Check sheet for the modelled part. Datum: model origin and axes. Units: mm. Give positions to 0.01 mm unless a question says otherwise; leave off trailing zeros. Order: outer loops, then holes, each group sorted by start corner. A loop starts at its lowest first (then second) coordinate and runs counter-clockwise, first axis right, second up.
```python
from build123d import *

# Parameters (mm, degrees)
EXTRUDE_1_DEPTH      = 3
EXTRUDE_1_DEPTH_BACK = 6
SKETCH_2_R           = 60
SKETCH_5_R           = 4
EXTRUDE_2_DEPTH      = 112
SKETCH_6_R           = 4
EXTRUDE_3_DEPTH      = 112
SKETCH_7_R           = 13
CUT_EXTRUDE_2_DEPTH  = 20
SKETCH_14_W          = 26
SKETCH_14_H          = 65
CUT_EXTRUDE_3_DEPTH  = 10


with BuildPart() as part:
    # 草图2 → 凸台-拉伸1 (new, two sides: drawn at the far end of the back side and taken through both)
    with BuildSketch(Plane.XY.offset(-EXTRUDE_1_DEPTH_BACK)):
        Circle(SKETCH_2_R)
    extrude(amount=EXTRUDE_1_DEPTH + EXTRUDE_1_DEPTH_BACK)

    # 草图5 → 凸台-拉伸2 (add)
    with BuildSketch(Plane(origin=(0, 0, -6), x_dir=(-1, 0, 0), z_dir=(0, 0, -1))):
        with Locations(Location((0, 50, 0), (0, 0, 180))):
            Circle(SKETCH_5_R)
    extrude(amount=EXTRUDE_2_DEPTH)

    # 草图6 → 凸台-拉伸3 (add)
    with BuildSketch(Plane(origin=(0, 0, -6), x_dir=(-1, 0, 0), z_dir=(0, 0, -1))):
        with Locations(Location((-44.655818583, -22.491284238, 0), (0, 0, 180))):
            Circle(SKETCH_6_R)
        with Locations(Location((41.95168902, -27.203966409, 0), (0, 0, 180))):
            Circle(SKETCH_6_R)
    extrude(amount=EXTRUDE_3_DEPTH)

    # 草图7 → 切除-拉伸2 (cut)
    with BuildSketch(Plane.XY.offset(3)):
        Circle(SKETCH_7_R)
    extrude(amount=-CUT_EXTRUDE_2_DEPTH, mode=Mode.SUBTRACT)

    # 草图14 → 切除-拉伸3 (cut)
    with BuildSketch(Plane.XY.offset(3)):
        with Locations((0, -32.5)):
            Rectangle(SKETCH_14_W, SKETCH_14_H)
    extrude(amount=-CUT_EXTRUDE_3_DEPTH, mode=Mode.SUBTRACT)


solid = part.part
```
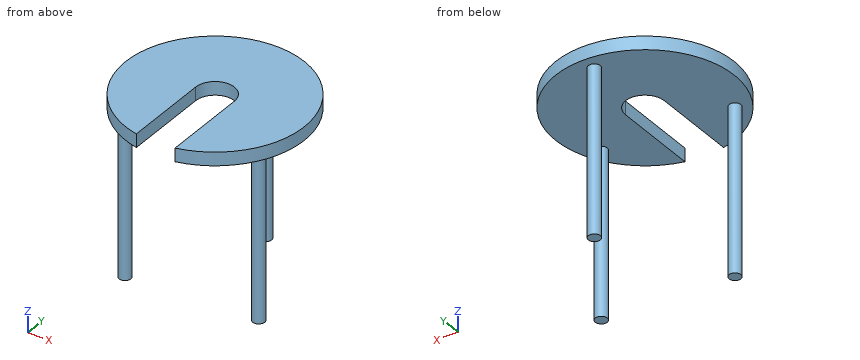
(1) Sectioned sample at C-C (y = 50). Enter the section's corners in (x, z).
(2) Sectioned sample at D-D (z = -4). Enter the section's corners in (x, y), plus the area to 3 significant figures.
(3) Sectioned sample at A-A (x = 0). Enter the section's corners in (y, z).
(4) Go/stop test with flat-tipped pins: P1, Ø3, axis at x = 4, z = -75.5, coming from the -Y side; P2, Ø2.5, axis at y = -44, z = -1.5, coming from the +X side; P3, Ø5, axis at x = -45.5, y = 8, coming from the -Z side. Record where each tip stops, or that it passes through.
(5) Sectioned sample at B-B (z = -47.5). Enter the section's corners in (x, y).
(6) Thickness scan on L1, parallel to Y at x = 0.5, z = -16; L2, parallel to Z at x = 6.5, y = 43; L3, parallel to X at y = 29, z = -2. Record the ranges inside material, lowest first.
Values follow:
1. outline: (-33.17, -6) - (-4, -6) - (-4, -118) - (4, -118) - (4, -6) - (33.17, -6) - (33.17, 3) - (-33.17, 3) - close
2. outline: (-13, -58.57) - (-13, 0) arc R13 cw to (13, 0) - (13, -58.57) arc R60 ccw (long way) to start
2. area: 9,500 mm2
3. outline: (13, -6) - (46, -6) - (46, -118) - (54, -118) - (54, -6) - (60, -6) - (60, 3) - (13, 3) - close
4. P1: stops at y = 46.88
4. P2: stops at x = 42.1
4. P3: stops at z = -6
5. outline: circle Ø8 at (-41.95, -27.2); circle Ø8 at (0, 50); circle Ø8 at (44.66, -22.49)
6. L1: y = 46.03 to 53.97
6. L2: z = -6 to 3
6. L3: x = -52.53 to 52.53
